from build123d import *

# Parameters (mm, degrees)
SKETCH1_R            = 35
BOSS_EXTRUDE1_DEPTH  = 1.5
M3_CLEARANCE_HOLE1_D = 3.4
FILLET1_R            = 10


with BuildPart() as part:
    # Sketch1 → Boss-Extrude1 (new, symmetric)
    with BuildSketch(Plane.XY):
        with BuildLine():
            Line((-63, 20), (-37.5, 20))
            ThreePointArc((-37.5, 20), (0, 42.5), (37.5, 20))
            Line((37.5, 20), (63, 20))
            Line((63, 20), (63, -20))
            Line((63, -20), (37.5, -20))
            ThreePointArc((37.5, -20), (0, -42.5), (-37.5, -20))
            Line((-37.5, -20), (-63, -20))
            Line((-63, -20), (-63, 20))
        make_face()
        Circle(SKETCH1_R, mode=Mode.SUBTRACT)
    extrude(amount=BOSS_EXTRUDE1_DEPTH, both=True)

    # M3 Clearance Hole1 (through all)
    with Locations(Plane.XY.offset(1.5)):
        with Locations((-58, 12.5), (-58, -12.5)):
            m3_clearance_hole1 = Hole(M3_CLEARANCE_HOLE1_D / 2)

    # Mirror1: M3 Clearance Hole1 across plane
    add(m3_clearance_hole1.mirror(Plane(origin=(0, 0, 0), x_dir=(0, 0, 1), z_dir=(1, 0, 0))), mode=Mode.SUBTRACT)

    # Fillet1
    fillet1_edges = [part.edges().sort_by_distance(p)[0] for p in [
        (37.5, 20, 0),
        (37.5, -20, 0),
        (-37.5, -20, 0),
        (-37.5, 20, 0),
    ]]
    fillet(fillet1_edges, radius=FILLET1_R)


solid = part.part
Read the model definition and answer for the solid it produces. Units are mm, in the model's axes. A direction names the side the tool comes from. Give positions to 0.01 mm unless a question says otherwise; leave off trailing zeros. Write each loop counter-clockwise with the first axis right and the second up, starting at its lowest first coordinate (ties: lowest second). Pieces come first, ordered by that corner, then holes. Notation, with made-up numbers: (-10, 22) -> (39, 22) arc R17 cw to (39, 41) -> close; hole circle Ø4 at (-26.75, 39). An arc over 180 degrees is marked (long way). Answer as a JSON object with one key per item and string values. Group by question number.
1) Each of these flat-tipped pins is pushed along its axis until it touches: P1, Ø3, axis at x = 58, y = 12.5, coming from the +Z side; P2, Ø1, axis at y = 28.5, z = -1, coming from the -X side; P3, Ø1.5, axis at x = 53, z = 0, coming from the -Y side. Where does it stop, or does it pass through?
2) Find section C-C (y = 29.5). Write down the section's boundary in (x, z).
3) Consider L1, parallel to Y at x = 58, z = 0.4; L2, parallel to Y at x = 0, z = -0.1; L3, parallel to Y at x = 27.5, z = 0. Determine where each line is inside the solid, lowest interval first. Write a range as from..to.
4) Find section B-B (z = -0.2). Write down the section's boundary in (x, y), and give its area (3 significant figures).
5) Find section D-D (x = 58). Write down the section's boundary in (y, z), and give its area (3 significant figures).
6) A tool of negligible diameter and unlimited length cuts with its end or side. For faces 1 (the flat face through (53, 20, 0)), 2 (the flat face through (-53, -20, 0)), 3 (the flat face through (-53, 20, 0)), from which of +Z, -Z, +X, -X, +Y, -Y can it reach the whole face along a straight path? Write none if from no direction.
7) The mould has two halves that part along Y. Classify faces 4 (the cylindrical face through (-56.3, -12.43, -0.02)), 5 (the cylindrical face through (-38.515, 21.105, -0.021)), 6 (the flat face through (63, 0, 0)): +Y half, -Y half, draft (parallel to the pull), parting line (faces both ways), or undercut.
8) Find section A-A (x = 0). Write down the section's boundary in (y, z).
Values follow:
{
 "1": {"P1": "passes through", "P2": "stops at x = -31.97", "P3": "stops at y = -20"},
 "2": {"outline": "(-30.59, -1.5) -> (-18.83, -1.5) -> (-18.83, 1.5) -> (-30.59, 1.5) -> close; (18.83, -1.5) -> (30.59, -1.5) -> (30.59, 1.5) -> (18.83, 1.5) -> close"},
 "3": {"L1": "y = -20..-14.2, -10.8..10.8, 14.2..20", "L2": "y = -42.5..-35, 35..42.5", "L3": "y = -32.4..-21.65, 21.65..32.4"},
 "4": {"outline": "(-63, -20) -> (-43.08, -20) arc R10 cw to (-34.88, -24.29) arc R42.5 ccw to (34.88, -24.29) arc R10 cw to (43.08, -20) -> (63, -20) -> (63, 20) -> (43.08, 20) arc R10 cw to (34.88, 24.29) arc R42.5 ccw to (-34.88, 24.29) arc R10 cw to (-43.08, 20) -> (-63, 20) -> close; hole circle Ø3.4 at (-58, -12.5); hole circle Ø3.4 at (-58, 12.5); hole circle Ø70 at (0, 0); hole circle Ø3.4 at (58, -12.5); hole circle Ø3.4 at (58, 12.5)", "area": "3,580 mm2"},
 "5": {"outline": "(-20, -1.5) -> (-14.2, -1.5) -> (-14.2, 1.5) -> (-20, 1.5) -> close; (-10.8, -1.5) -> (10.8, -1.5) -> (10.8, 1.5) -> (-10.8, 1.5) -> close; (14.2, -1.5) -> (20, -1.5) -> (20, 1.5) -> (14.2, 1.5) -> close", "area": "99.6 mm2"},
 "6": {"face 1": "+Z, -Z, +X, +Y", "face 2": "+Z, -Z, -X, -Y", "face 3": "+Z, -Z, -X, +Y"},
 "7": {"face 4": "undercut", "face 5": "+Y half", "face 6": "draft"},
 "8": {"outline": "(-42.5, -1.5) -> (-35, -1.5) -> (-35, 1.5) -> (-42.5, 1.5) -> close; (35, -1.5) -> (42.5, -1.5) -> (42.5, 1.5) -> (35, 1.5) -> close"}
}
